Read the model definition and answer for the solid it produces. Units are mm, in the model's axes. Coordinates: 2 decimals unless noted, no trailing zeros. Order: outer loops, then holes, each group sorted by start corner. A loop starts at its lowest first (then second) coordinate and runs counter-clockwise, first axis right, second up. Notation, with made-up numbers: (89.5, -9) - (139.5, -9) arc R18 ccw to (139.5, 15) - close; hole circle Ø2 at (79.5, -14.5). An arc over 180 degrees is marked (long way). Use one line per item in the form item = value. Start each with the question number.
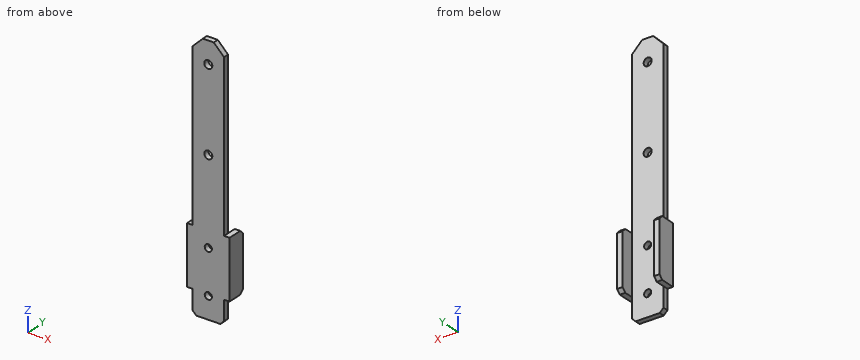
from build123d import *

# Parameters (mm, degrees)
SKETCH006_W              = 8.6
SKETCH006_H              = 70
SKETCH006_R              = 1.1
SKETCH006_R_2            = 0.975
PAD005_DEPTH             = 1.5
SKETCH007_W              = 1.5
SKETCH007_H              = 16
PAD006_DEPTH             = 5
CHAMFER001_SIZE          = 2.8
CHAMFER002_SIZE          = 1
CLONE002_PLACEMENT_ANGLE = 180


with BuildPart() as part:
    # Sketch006 (on Face74 of Binder003) → Pad005 (new body)
    with BuildSketch(Plane(origin=(-7.1e-05, -19.1, 0.000123), x_dir=(1, -4e-06, 0), z_dir=(-4e-06, -1, 6e-06))):
        with Locations((12.106057, -34.481964)):
            Rectangle(SKETCH006_W, SKETCH006_H)
        with Locations((12.106057, -5.481964)):
            Circle(SKETCH006_R, mode=Mode.SUBTRACT)
        with Locations((12.106057, -28.152043)):
            Circle(SKETCH006_R, mode=Mode.SUBTRACT)
        with Locations((12.106057, -51.481964)):
            Circle(SKETCH006_R_2, mode=Mode.SUBTRACT)
        with Locations((12.106057, -63.481964)):
            Circle(SKETCH006_R_2, mode=Mode.SUBTRACT)
    extrude(amount=PAD005_DEPTH)

    # Sketch007 (on Face9 of Pad005) → Pad006 (join)
    with BuildSketch(Plane(origin=(-7.1e-05, -19.1, 0.000123), x_dir=(-1, 4e-06, 0), z_dir=(4e-06, 1, -6e-06))):
        with Locations((-17.156057, -55.081964)):
            Rectangle(SKETCH007_W, SKETCH007_H)
        with Locations((-7.056057, -55.081964)):
            Rectangle(SKETCH007_W, SKETCH007_H)
    extrude(amount=-PAD006_DEPTH)

    # Chamfer001
    chamfer001_edges = [part.edges().sort_by_distance(p)[0] for p in [
        (16.405983, -19.850058, 0.518165),
        (7.805983, -19.850026, 0.518165),
    ]]
    chamfer(chamfer001_edges, length=CHAMFER001_SIZE)

    # Chamfer002
    chamfer002_edges = [part.edges().sort_by_distance(p)[0] for p in [
        (17.155967, -24.100368, -47.081808),
        (17.155967, -24.100471, -63.081808),
        (7.055967, -24.100433, -63.081808),
        (7.055967, -24.10033, -47.081808),
        (16.405983, -19.850509, -69.481835),
        (7.805983, -19.850477, -69.481835),
    ]]
    chamfer(chamfer002_edges, length=CHAMFER002_SIZE)


with BuildPart() as part_1:
    # Clone002 placement: moved
    add(part.part.moved(Location((6.2, 0, 10.4))).rotate(Axis((6.2, 0, 10.4), (0, 0, 1)), CLONE002_PLACEMENT_ANGLE))


solid = part_1.part
Q1. A cutting plane is placed at A-A (y = 22.15). Give the vertices of the cut face in (x, z).
Q2. Consider probe 1 along X at (y, z) = (23.8, -38); probe 2 along Y at (x, z) = (-9.25, -35.5); probe 3 along X at (y, z) = (19.7, -35.5). Determine where each line is inside the solid, lowest interval first.
Q3. A cutting plane is placed at B-B (x = -1). Give the vertices of the cut face in (y, z), then the cut area to 3 significant figures.
Q4. A cutting plane is placed at D-D (x = -3.75). Give the vertices of the cut face in (y, z).
Q5. Given P1, Ø0.5, axis at y = 20, z = -10.5, coming from the +X side; P2, Ø1.2, axis at y = 20, z = -6, coming from the -X side; P3, Ø0.5, axis at x = -1, y = 20, coming from the +Z side, each flat-ended and moving along its own axis, determine where each tip first touches the part or whether it passes through.
Q6. A cutting plane is placed at C-C (z = -46). Give the vertices of the cut face in (x, y).
Result sheet:
q1.outline = (-11.71, -52.68) - (-10.21, -52.68) - (-10.21, -36.68) - (-11.71, -36.68) - close; (-1.61, -52.68) - (-0.11, -52.68) - (-0.11, -36.68) - (-1.61, -36.68) - close
q2.probe_1 = -11.71 to -10.21, -1.61 to -0.11
q2.probe_2 = 19.1 to 20.6
q2.probe_3 = -10.21 to -1.61
q3.outline = (19.1, -52.68) - (23.1, -52.68) - (24.1, -51.68) - (24.1, -37.68) - (23.1, -36.68) - (19.1, -36.68) - close
q3.area = 79.0 mm^2
q4.outline = (19.1, -59.08) - (20.6, -59.08) - (20.6, 10.26) - (19.1, 10.26) - close
q5.P1 = -1.61
q5.P2 = -10.21
q5.P3 = -36.68
q6.outline = (-11.71, 19.1) - (-0.11, 19.1) - (-0.11, 24.1) - (-1.61, 24.1) - (-1.61, 20.6) - (-10.21, 20.6) - (-10.21, 24.1) - (-11.71, 24.1) - close
